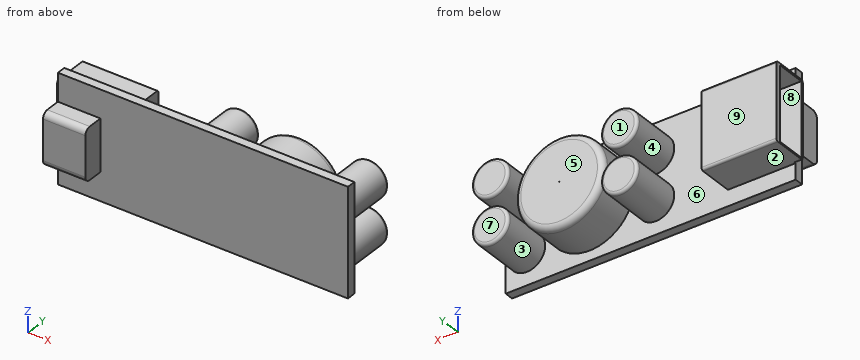
```python
from build123d import *

# Parameters (mm, degrees)
SKETCH_1_W          = 49.2
SKETCH_1_H          = 18.3
EXTRUDE_361_DEPTH   = 1.5
SKETCH_3_W          = 12.7
SKETCH_3_H          = 13.1
EXTRUDE_2_DEPTH     = 6.2
SKETCH_4_W          = 7.2
SKETCH_4_H          = 8.8
EXTRUDE_3_DEPTH     = 3.5
FILLET_2_R          = 1
FILLET_3_R          = 0.4
SKETCH_5_R          = 3.1
EXTRUDE_4_DEPTH     = 8.7
FILLET_5_R          = 0.5
SKETCH_6_R          = 7.5
SKETCH_6_R_2        = 0.053550992
EXTRUDE_5_DEPTH     = 7.2
FILLET_6_R          = 1
SKETCH_7_W          = 12.5
SKETCH_7_H          = 5
CUT_EXTRUDE_1_DEPTH = 10.2
FILLET_7_R          = 0.4


with BuildPart() as part:
    # Эскиз1 → Extrude 361 (new body)
    with BuildSketch(Plane(origin=(0, 0, 0), x_dir=(1, 0, 0), z_dir=(0, 1, 0))):
        Rectangle(SKETCH_1_W, SKETCH_1_H)
    extrude(amount=EXTRUDE_361_DEPTH)

    # Эскиз3 → Бобышка-Вытянуть2 (add)
    with BuildSketch(Plane(origin=(0, 1.5, 0), x_dir=(1, 0, 0), z_dir=(0, 1, 0))):
        with Locations((-19.45, -0.1)):
            Rectangle(SKETCH_3_W, SKETCH_3_H)
    extrude(amount=EXTRUDE_2_DEPTH)

    # Эскиз4 → Бобышка-Вытянуть3 (add)
    with BuildSketch(Plane.XZ):
        with Locations((-21, 0)):
            Rectangle(SKETCH_4_W, SKETCH_4_H)
    extrude(amount=EXTRUDE_3_DEPTH)

    # Скругление2
    fillet_2_edges = [part.edges().sort_by_distance(p)[0] for p in [
        (-21, -3.5, 4.4),
        (-21, -3.5, -4.4),
    ]]
    fillet(fillet_2_edges, radius=FILLET_2_R)

    # Скругление3
    fillet_3_edges = [part.edges().sort_by_distance(p)[0] for p in [
        (-19.45, 7.7, -6.45),
        (-19.45, 7.7, 6.65),
    ]]
    fillet(fillet_3_edges, radius=FILLET_3_R)

    # Эскиз5 → Бобышка-Вытянуть4 (add)
    with BuildSketch(Plane(origin=(0, 1.5, 0), x_dir=(1, 0, 0), z_dir=(0, 1, 0))):
        with Locations(Location((21, 3.85, 0), (0, 0, 270))):
            Circle(SKETCH_5_R)
        with Locations(Location((21, -3.85, 0), (0, 0, 270))):
            Circle(SKETCH_5_R)
        with Locations(Location((-0.9, -3.85, 0), (0, 0, 270))):
            Circle(SKETCH_5_R)
        with Locations(Location((-0.9, 3.85, 0), (0, 0, 270))):
            Circle(SKETCH_5_R)
    extrude(amount=EXTRUDE_4_DEPTH)

    # Скругление5
    fillet_5_edges = [part.edges().sort_by_distance(p)[0] for p in [
        (21, 10.2, -6.95),
        (21, 10.2, 0.75),
        (-0.9, 10.2, 0.75),
        (-0.9, 10.2, -6.95),
    ]]
    fillet(fillet_5_edges, radius=FILLET_5_R)

    # Эскиз6 → Бобышка-Вытянуть5 (add)
    with BuildSketch(Plane(origin=(0, 1.5, 0), x_dir=(1, 0, 0), z_dir=(0, 1, 0))):
        with Locations(Location((10.324402455, 0, 0), (0, 0, 270))):
            Circle(SKETCH_6_R)
        with Locations(Location((10.324402455, 0, 0), (0, 0, 270))):
            Circle(SKETCH_6_R_2, mode=Mode.SUBTRACT)
    extrude(amount=EXTRUDE_5_DEPTH)

    # Скругление6
    fillet_6_edges = [part.edges().sort_by_distance(p)[0] for p in [
        (10.324402455, 8.7, -7.5),
    ]]
    fillet(fillet_6_edges, radius=FILLET_6_R)

    # Эскиз7 → Вырез-Вытянуть1 (cut)
    with BuildSketch(Plane.ZY.offset(25.8)):
        with Locations((0.078486032, 4.347326387)):
            Rectangle(SKETCH_7_W, SKETCH_7_H)
    extrude(amount=-CUT_EXTRUDE_1_DEPTH, mode=Mode.SUBTRACT)

    # Скругление7
    fillet_7_edges = [part.edges().sort_by_distance(p)[0] for p in [
        (-25.2, 1.5, -6.45),
        (-25.2, 1.5, 6.65),
    ]]
    fillet(fillet_7_edges, radius=FILLET_7_R)


solid = part.part
```
Geometry: final body of the model. Coordinates: model frame, mm. Face numbers are marked on the shaded views. A direction names the side the tool comes from. Coordinates: 2 decimals unless noted, no trailing zeros. Order: outer loops, then holes, each group sorted by start corner. A loop starts at its lowest first (then second) coordinate and runs counter-clockwise, first axis right, second up. Notation, with made-up numbers: (5.25, 19.25) -> (19.25, 19.25) arc R12 cw to (19.25, 25.25) -> close; hole circle Ø3 at (64.5, 66.5). An arc over 180 degrees is marked (long way). Answer in a Markdown table with one row per item.
Item 1: Ray query, L1, parallel to Y at x = -18, z = 0.25; L2, parallel to X at y = 2.5, z = 3; L3, parallel to Z at x = -14, y = 6. Return the intervals inside material, ascending.
Return value:
| item | result |
|---|---|
| L1 | y = -3.5 to 1.85, 6.85 to 7.7 |
| L2 | x = -15.6 to -13.1, -3.88 to 2.08, 3.45 to 17.2, 18.02 to 23.98 |
| L3 | z = -6.45 to 6.65 |
Item 2: Section A-A on y = 8.25. Output: boundary loops of the cut face in (x, z).
Return value:
| item | result |
|---|---|
| outline | circle Ø6.2 at (-0.9, -3.85); circle Ø6.2 at (-0.9, 3.85); circle Ø14.67 at (10.32, 0); circle Ø6.2 at (21, -3.85); circle Ø6.2 at (21, 3.85); hole circle Ø0.11 at (10.32, 0) |
Item 3: Contact query for flat-ended pins moving along their axis: P1, Ø4.5, axis at x = -20, y = 4.5, coming from the +Z side; P2, Ø2, axis at x = -22.5, y = -1.5, coming from the +Z side; P3, Ø8, axis at x = -11.5, z = 0, coming from the -Y side. Output: stop coordinate, or through.
Return value:
| item | result |
|---|---|
| P1 | stops at z = 6.65 |
| P2 | stops at z = 4.4 |
| P3 | stops at y = 0 |
Item 4: Draft query along Z for the marked faces 1, 2, 3 and 4. Return one class per face: released by +Z, released by -Z, zero draft, split by the parting line, or undercut.
Return value:
| item | result |
|---|---|
| face 1 | zero draft |
| face 2 | released by -Z |
| face 3 | undercut |
| face 4 | undercut |
Item 5: Access query for the marked faces 5, 6, 7, 8 and 9. Directions: +Z, -Z, +X, -X, +Y, -Y. A direction counts if a zero-diameter tool reaches every point of the face in a straight line with its end or side. Return the directions, or none.
Return value:
| item | result |
|---|---|
| face 5 | +Z, -Z, +Y |
| face 6 | +Y |
| face 7 | +Z, -Z, +X, -X, +Y |
| face 8 | -X |
| face 9 | +Z, -Z, -X, +Y |
Item 6: Section B-B on x = -0.9. Output: boundary loops of the cut face in (y, z), plus the area to 3 significant figures.
Return value:
| item | result |
|---|---|
| outline | (0, -9.15) -> (1.5, -9.15) -> (1.5, -6.95) -> (9.7, -6.95) arc R0.5 ccw to (10.2, -6.45) -> (10.2, -1.25) arc R0.5 ccw to (9.7, -0.75) -> (1.5, -0.75) -> (1.5, 0.75) -> (9.7, 0.75) arc R0.5 ccw to (10.2, 1.25) -> (10.2, 6.45) arc R0.5 ccw to (9.7, 6.95) -> (1.5, 6.95) -> (1.5, 9.15) -> (0, 9.15) -> close |
| area | 135 mm² |
Item 7: Section C-C on y = 5.75. Output: boundary loops of the cut face in (x, z).
Return value:
| item | result |
|---|---|
| outline | (-25.8, -6.45) -> (-13.1, -6.45) -> (-13.1, 6.65) -> (-25.8, 6.65) -> (-25.8, 6.33) -> (-15.6, 6.33) -> (-15.6, -6.17) -> (-25.8, -6.17) -> close; circle Ø6.2 at (-0.9, -3.85); circle Ø6.2 at (-0.9, 3.85); circle Ø15 at (10.32, 0); circle Ø6.2 at (21, -3.85); circle Ø6.2 at (21, 3.85); hole circle Ø0.11 at (10.32, 0) |
